from build123d import *

# Parameters (mm, degrees)
SKETCH1_R           = 2.794
BOSS_EXTRUDE1_DEPTH = 3.81
SKETCH3_R           = 4.445
CUT_EXTRUDE1_DEPTH  = 2.54
BOSS_EXTRUDE2_START = 2.54
SKETCH4_R           = 5.334
SKETCH4_R_2         = 2.794
BOSS_EXTRUDE2_DEPTH = 2.54
FILLET2_R           = 0.762


with BuildPart() as part:
    # Sketch1 → Boss-Extrude1 (new body)
    with BuildSketch(Plane(origin=(0, 0, 0), x_dir=(1, 0, 0), z_dir=(0, 1, 0))):
        with BuildLine():
            ThreePointArc((11.341805556, 5.714319447), (5.715, 0), (11.341805556, -5.714319447))
            ThreePointArc((11.341805556, -5.714319447), (-12.7, 0), (11.341805556, 5.714319447))
        make_face()
        with Locations(Location((0, 0, 0), (0, 0, 90))):
            Circle(SKETCH1_R, mode=Mode.SUBTRACT)
    extrude(amount=BOSS_EXTRUDE1_DEPTH)

    # Sketch3 → Cut-Extrude1 (cut)
    with BuildSketch(Plane(origin=(0, 3.81, 0), x_dir=(1, 0, 0), z_dir=(0, 1, 0))):
        with Locations(Location((0, 0, 0), (0, 0, 270))):
            Circle(SKETCH3_R)
    extrude(amount=-CUT_EXTRUDE1_DEPTH, mode=Mode.SUBTRACT)

    # Sketch4 → Boss-Extrude2 (add)
    with BuildSketch(Plane.XZ.offset(BOSS_EXTRUDE2_START)):
        with Locations(Location((0, 0, 0), (0, 0, 90))):
            Circle(SKETCH4_R)
        with Locations(Location((0, 0, 0), (0, 0, 270))):
            Circle(SKETCH4_R_2, mode=Mode.SUBTRACT)
    extrude(amount=-BOSS_EXTRUDE2_DEPTH)

    # Fillet2
    fillet2_edges = [part.edges().sort_by_distance(p)[0] for p in [
        (5.715, 3.81, 0),
        (5.715, 0, 0),
        (11.341805556, 1.905, 5.714319447),
        (11.341805556, 1.905, -5.714319447),
    ]]
    fillet(fillet2_edges, radius=FILLET2_R)


solid = part.part
Could you check a few things on this model? Use its own coordinates, in mm. A direction names the side the tool comes from. Coordinates: 2 decimals unless noted, no trailing zeros. Write each loop counter-clockwise with the first axis right and the second up, starting at its lowest first coordinate (ties: lowest second). Pieces come first, ordered by that corner, then holes. Notation, with made-up numbers: (19.25, -24) - (72.25, -24) arc R11 ccw to (72.25, -6) - close; hole circle Ø7 at (47, -1.75). An arc over 180 degrees is marked (long way). Put each result on its own line as item: value. Start each with the question number.
Q1. I want a section at A-A on x = 0. Write out the boundary of the cut face in (y, z) (3 decimals).
Q2. Please list where these lines run through material, in increasing order: L1, parallel to X at y = 2.25, z = 0 (3 decimals); L2, parallel to X at y = -1.5, z = 0; L3, parallel to Y at x = -6.75, z = 9.25.
Q3. Thinking about a two-plate mould opening in X: for faces 1 (the cylindrical face through (3.25, -1.29, -4.23)), 2 (the cylindrical face through (5.716, 1.823, -0.109)), 3 (the flat face through (-3, 1.27, 0)), which applies, pulls with the +X half, pulls with the -X half, needs draft (parallel to the pull), parting line crosses it, or undercut?
Q4. I want a section at C-C on x = -7. Write out the boundary of the cut face in (y, z), plus the area to 3 significant figures.
Q5. Which directions (+Z, -Z, +X, -X, +Y, -Y) give clear straight access to the entire face, cutting with the end or side of a thin tool? Please do faces 4 (the flat face through (-6, 3.81, 0)), 5 (the cylindrical face through (-4.34, 2.56, -0.96)).
Q6. I want a section at B-B on z = 9.75. Write out the boundary of the cut face in (x, y), plus the area to 3 significant figures.
Q7. I'm going to push flat-ended pins straight in: P1, Ø10, axis at x = -1.5, z = -1.5, coming from the +Y side; P2, Ø2, axis at x = -3.5, y = 1.5, coming from the -Z side; P3, Ø1.5, axis at y = 2.5, z = 1.5, coming from the -X side. Where does each tip first touch, or does it pass through?
Checks:
1. outline: (-2.54, -5.334) - (0, -5.334) - (0, -12.7) - (3.81, -12.7) - (3.81, -4.445) - (1.27, -4.445) - (1.27, -2.794) - (-2.54, -2.794) - close; (-2.54, 2.794) - (1.27, 2.794) - (1.27, 4.445) - (3.81, 4.445) - (3.81, 12.7) - (0, 12.7) - (0, 5.334) - (-2.54, 5.334) - close
2. L1: -12.7 to -4.445, 4.445 to 5.715
2. L2: -5.33 to -2.79, 2.79 to 5.33
2. L3: 0 to 3.81
3. face 1: parting line crosses it
3. face 2: pulls with the +X half
3. face 3: undercut
4. outline: (0, -10.6) - (3.81, -10.6) - (3.81, 10.6) - (0, 10.6) - close
4. area: 80.7 mm²
5. face 4: +Z, -Z, +X, -X, +Y
5. face 5: +Y
6. outline: (-8.14, 0) - (8.14, 0) - (8.14, 3.81) - (-8.14, 3.81) - close
6. area: 62.0 mm²
7. P1: y = 3.81
7. P2: z = -12.45
7. P3: x = -12.68
